from build123d import *

# Parameters (mm, degrees)
CORTE_EXTRUS_O1_DEPTH = 2


with BuildPart() as part:
    # Esboço1 → Revolução1 (revolve)
    with BuildSketch(Plane.XY):
        Polygon((1.65, 0), (5.5, 0), (5.5, 2), (4, 3.5), (5.5, 5), (5.5, 7), (1.65, 7), align=None)
    revolve(axis=Axis((0, 0, 0), (0, 1, 0)))

    # Esboço2 → Corte-extrusão1 (cut)
    with BuildSketch(Plane(origin=(0, 7, 0), x_dir=(1, 0, 0), z_dir=(0, 1, 0))):
        Polygon((3.233161507, 0), (1.616580754, 2.8), (-1.616580754, 2.8), (-3.233161507, 0), (-1.616580754, -2.8), (1.616580754, -2.8), align=None)
    extrude(amount=-CORTE_EXTRUS_O1_DEPTH, mode=Mode.SUBTRACT)


solid = part.part
Check sheet for the modelled part. Datum: model origin and axes. Units: mm. A direction names the side the tool comes from. Give positions to 0.01 mm unless a question says otherwise; leave off trailing zeros. Write each loop counter-clockwise with the first axis right and the second up, starting at its lowest first coordinate (ties: lowest second). Pieces come first, ordered by that corner, then holes. Notation, with made-up numbers: (75.25, 36.25) -> (94.25, 36.25) arc R36 ccw to (94.25, 70.25) -> close; hole circle Ø5 at (1, 27). An arc over 180 degrees is marked (long way). Use one line per item in the form item = value. Start each with the question number.
1. Go/stop test with flat-tipped pins: P1, Ø4, axis at y = 4.5, z = 3.5, coming from the -X side; P2, Ø3, axis at y = 4.5, z = -4, coming from the -X side; P3, Ø1, axis at x = -1, y = 6, coming from the -Z side; P4, Ø6, axis at x = 0.5, z = -1, coming from the +Y side. Record where each tip stops, or that it passes through.
2. Access from +Z, -Z, +X, -X, +Y, -Y to the whole of each face (thin tool, end or side, straight path). Record for faces 5 (the flat face through (0, 6, -2.8)), 6 (the cylindrical face through (-1.19, 6.01, 5.37)).
3. Section check B-B (y = 6.5). Record the cut outline in (x, z), and give its area (3 significant figures).
4. Thickness scan on line 1 along Z through (x, y) = (0, 1.1); line 2 along Z through (x, y) = (-2, 5.5). Record the ranges inside material, lowest first. Write a range as from..to.
5. Section check D-D (y = 3). Record the cut outline in (x, z).
6. Section check C-C (y = 0.5). Record the cut outline in (x, z).
7. Mould release check, pull along Z, two halves, no side actions. Record for faces 1 (the flat face through (-2.436, 6.014, 1.38)), 2 (the cylindrical face through (-1.216, 2.465, -1.115)), 3 (the flat face through (-3, 7, -1)), 4 (the cylindrical face through (-1.19, 1.01, 5.37)): pulls with the +Z half, pulls with the -Z half, needs draft (parallel to the pull), parting line crosses it, or undercut.
8. Section check A-A (x = 0). Record the cut outline in (y, z), and give its area (3 significant figures).
Conclusion:
q1.P1 = -5.27
q1.P2 = -4.85
q1.P3 = -5.48
q1.P4 = 7
q2.face_5 = +Y
q2.face_6 = +Y, -Y
q3.outline = circle Ø11 at (0, 0); hole (-3.23, 0) -> (-1.62, -2.8) -> (1.62, -2.8) -> (3.23, 0) -> (1.62, 2.8) -> (-1.62, 2.8) -> close
q3.area = 67.9 mm²
q4.line_1 = -5.5..-1.65, 1.65..5.5
q4.line_2 = -5.12..-2.14, 2.14..5.12
q5.outline = circle Ø9 at (0, 0); hole circle Ø3.3 at (0, 0)
q6.outline = circle Ø11 at (0, 0); hole circle Ø3.3 at (0, 0)
q7.face_1 = undercut
q7.face_2 = undercut
q7.face_3 = needs draft
q7.face_4 = parting line crosses it
q8.outline = (0, -5.5) -> (2, -5.5) -> (3.5, -4) -> (5, -5.5) -> (7, -5.5) -> (7, -2.8) -> (5, -2.8) -> (5, -1.65) -> (0, -1.65) -> close; (0, 1.65) -> (5, 1.65) -> (5, 2.8) -> (7, 2.8) -> (7, 5.5) -> (5, 5.5) -> (3.5, 4) -> (2, 5.5) -> (0, 5.5) -> close
q8.area = 44.8 mm²
